Model file for the job. Use its own axes, mm. Coordinates: 2 decimals unless noted, no trailing zeros. Write each loop counter-clockwise with the first axis right and the second up, starting at its lowest first coordinate (ties: lowest second). Pieces come first, ordered by that corner, then holes. Notation, with made-up numbers: M -5.75,-1.5 L 15.25,-1.5 A17 ccw 15.25,8.5 Z; hole C 50.25,-0.75 d3. An arc over 180 degrees is marked long. Answer in a Markdown table with one row per item. Add a question column.
```python
from build123d import *

# Parameters (mm, degrees)
SKETCH_1_W          = 27
SKETCH_1_H          = 25
EXTRUDE_1_DEPTH     = 1.5
SKETCH_2_R          = 0.45
SKETCH_2_W          = 0.6
SKETCH_2_H          = 0.4
SKETCH_2_W_2        = 0.7
SKETCH_2_H_2        = 0.7
CUT_EXTRUDE_1_DEPTH = 19.459414942


with BuildPart() as part:
    # Эскиз1 → Бобышка-Вытянуть1 (new body)
    with BuildSketch(Plane(origin=(0, 0, 0), x_dir=(1, 0, 0), z_dir=(0, 1, 0))):
        Rectangle(SKETCH_1_W, SKETCH_1_H)
    extrude(amount=EXTRUDE_1_DEPTH)

    # Эскиз2 → Вырез-Вытянуть1 (cut, through all)
    with BuildSketch(Plane(origin=(0, 1.5, 0), x_dir=(1, 0, 0), z_dir=(0, 1, 0))):
        with Locations(Location((11.5, 9.9, 0), (0, 0, 270))):
            Circle(SKETCH_2_R)
        with Locations(Location((11.5, 7.36, 0), (0, 0, 270))):
            Circle(SKETCH_2_R)
        with Locations(Location((11.5, 4.82, 0), (0, 0, 270))):
            Circle(SKETCH_2_R)
        with Locations(Location((11.5, 2.28, 0), (0, 0, 270))):
            Circle(SKETCH_2_R)
        with Locations(Location((11.5, -0.26, 0), (0, 0, 270))):
            Circle(SKETCH_2_R)
        with Locations(Location((11.5, -2.8, 0), (0, 0, 270))):
            Circle(SKETCH_2_R)
        with Locations(Location((11.5, -5.34, 0), (0, 0, 270))):
            Circle(SKETCH_2_R)
        with Locations(Location((11.5, -7.88, 0), (0, 0, 270))):
            Circle(SKETCH_2_R)
        with Locations((-9.16, 9.8)):
            Rectangle(SKETCH_2_W, SKETCH_2_H)
        with Locations((-11.7, 9.8)):
            Rectangle(SKETCH_2_W, SKETCH_2_H)
        with Locations((-6.62, 9.8)):
            Rectangle(SKETCH_2_W, SKETCH_2_H)
        with Locations((-4.08, 9.8)):
            Rectangle(SKETCH_2_W, SKETCH_2_H)
        with Locations((-1.54, 9.8)):
            Rectangle(SKETCH_2_W, SKETCH_2_H)
        with Locations((1, 9.8)):
            Rectangle(SKETCH_2_W, SKETCH_2_H)
        with Locations((3.54, 9.8)):
            Rectangle(SKETCH_2_W, SKETCH_2_H)
        with Locations((6.08, 9.8)):
            Rectangle(SKETCH_2_W, SKETCH_2_H)
        with Locations((-9.547856055, -10.59636646)):
            Rectangle(SKETCH_2_W_2, SKETCH_2_H_2)
        with Locations((-7.007856055, -10.59636646)):
            Rectangle(SKETCH_2_W_2, SKETCH_2_H_2)
        with Locations((-4.467856055, -10.59636646)):
            Rectangle(SKETCH_2_W_2, SKETCH_2_H_2)
        with Locations((-1.927856055, -10.59636646)):
            Rectangle(SKETCH_2_W_2, SKETCH_2_H_2)
        with Locations((0.612143945, -10.59636646)):
            Rectangle(SKETCH_2_W_2, SKETCH_2_H_2)
        with Locations((3.152143945, -10.59636646)):
            Rectangle(SKETCH_2_W_2, SKETCH_2_H_2)
        with Locations((5.692143945, -10.59636646)):
            Rectangle(SKETCH_2_W_2, SKETCH_2_H_2)
        with Locations((8.232143945, -10.59636646)):
            Rectangle(SKETCH_2_W_2, SKETCH_2_H_2)
        with Locations((-12.087856055, -10.59636646)):
            Rectangle(SKETCH_2_W_2, SKETCH_2_H_2)
    extrude(amount=-CUT_EXTRUDE_1_DEPTH, mode=Mode.SUBTRACT)


solid = part.part
```
1) Drill centre lines: probe 1 along X at (y, z) = (1.05, 0.26); probe 2 along Z at (x, y) = (-11.5, 0.5); probe 3 along X at (y, z) = (0.5, 7.5). Where is each one in solid material? Low to high.
2) Slice it at A-A (z = 5.34). Give the cut face in (x, y).
3) Two-plate mould, pull along Z, no slides. Class faces 1 (the face through (11.88, 0.76, -4.58)), 2 (the face through (0, 1, 12.5)), 3 (the face through (11.946, 0.76, -7.419)), 4 (the face through (0, 0, 0)): released by +Z, released by -Z, zero draft, split by the parting line, or undercut.
4) Slice it at B-B (y = 0.4). Count the separate pieces of the cut face and the enclosed holes in it, then the cut area to 3 significant figures.
Ans:
| question | item | result |
|---|---|---|
| 1 | probe 1 | x = -13.5 to 11.05, 11.95 to 13.5 |
| 1 | probe 2 | z = -12.5 to -10, -9.6 to 12.5 |
| 1 | probe 3 | x = -13.5 to 11.26, 11.74 to 13.5 |
| 2 | outline | M -13.5,0 L 11.05,0 L 11.05,1.5 L -13.5,1.5 Z; M 11.95,0 L 13.5,0 L 13.5,1.5 L 11.95,1.5 Z |
| 3 | face 1 | undercut |
| 3 | face 2 | released by +Z |
| 3 | face 3 | undercut |
| 3 | face 4 | zero draft |
| 4 | separate pieces | 1 |
| 4 | enclosed holes | 25 |
| 4 | area | 664 mm2 |
